from build123d import *

# Parameters (mm, degrees)
ESBO_O1_W                = 95.625
ESBO_O1_H                = 63.75
RESSALTO_EXTRUS_O1_DEPTH = 50
RESSALTO_EXTRUS_O2_DEPTH = 100
CORTE_EXTRUS_O1_DEPTH    = 100
CORTE_EXTRUS_O2_DEPTH    = 169
RESSALTO_EXTRUS_O3_DEPTH = 5


with BuildPart() as part:
    # Esboço1 → Ressalto-extrusão1 (new body)
    with BuildSketch(Plane.XY):
        with BuildLine():
            Line((0, 0), (0, -110))
            ThreePointArc((0, -110), (60, -134.792027106), (120, -110))
            Line((120, -110), (120, 0))
            ThreePointArc((120, 0), (60, 24.792027106), (0, 0))
        make_face()
        with Locations((60, -55)):
            Rectangle(ESBO_O1_W, ESBO_O1_H, mode=Mode.SUBTRACT)
    extrude(amount=RESSALTO_EXTRUS_O1_DEPTH)

    # Esboço2 → Ressalto-extrusão2 (add)
    with BuildSketch(Plane(origin=(0, 0, 0), x_dir=(-1, 0, 0), z_dir=(0, 0, -1))):
        with BuildLine():
            Line((-125, 2.041525096), (-125, -112.041525096))
            ThreePointArc((-125, -112.041525096), (-60, -139.792027106), (5, -112.041525096))
            Line((5, -112.041525096), (5, 2.041525096))
            ThreePointArc((5, 2.041525096), (-60, 29.792027106), (-125, 2.041525096))
        make_face()
        with BuildLine():
            Line((0, 0), (0, -110))
            ThreePointArc((0, -110), (-60, -134.792027106), (-120, -110))
            Line((-120, -110), (-120, 0))
            ThreePointArc((-120, 0), (-60, 24.792027106), (0, 0))
        make_face(mode=Mode.SUBTRACT)
    extrude(amount=-RESSALTO_EXTRUS_O2_DEPTH)

    # Esboço3 → Corte-extrusão1 (cut)
    with BuildSketch(Plane.XY.offset(50)):
        with BuildLine():
            Line((0, 0), (0, -110))
            ThreePointArc((0, -110), (60, -134.792027106), (120, -110))
            Line((120, -110), (120, 0))
            ThreePointArc((120, 0), (60, 24.792027106), (0, 0))
        make_face()
    extrude(amount=-CORTE_EXTRUS_O1_DEPTH, mode=Mode.SUBTRACT)

    # Esboço4 → Corte-extrusão2 (cut)
    with BuildSketch(Plane(origin=(125, 0, 0), x_dir=(0, 0, -1), z_dir=(1, 0, 0))):
        Polygon((-50, -55), (-100, -17.994062777), (-100, -175.493521459), (-50, -175.493521459), align=None)
    extrude(amount=-CORTE_EXTRUS_O2_DEPTH, mode=Mode.SUBTRACT)

    # Esboço5 → Ressalto-extrusão3 (add)
    with BuildSketch(Plane(origin=(0, 0, 0), x_dir=(-1, 0, 0), z_dir=(0, 0, -1))):
        with BuildLine():
            Line((-125, 2.041525096), (-125, -112.041525096))
            ThreePointArc((-125, -112.041525096), (-60, -139.792027106), (5, -112.041525096))
            Line((5, -112.041525096), (5, 2.041525096))
            ThreePointArc((5, 2.041525096), (-60, 29.792027106), (-125, 2.041525096))
        make_face()
        with BuildLine():
            Line((-116, -1.68447334), (-116, -108.31552666))
            ThreePointArc((-116, -108.31552666), (-60, -130.792027106), (-4, -108.31552666))
            Line((-4, -108.31552666), (-4, -1.68447334))
            ThreePointArc((-4, -1.68447334), (-60, 20.792027106), (-116, -1.68447334))
        make_face(mode=Mode.SUBTRACT)
    extrude(amount=RESSALTO_EXTRUS_O3_DEPTH)


solid = part.part
Build history of the part. All positions in model axes, mm. A direction names the side the tool comes from. Round coordinates to 2 decimals unless told otherwise and drop trailing zeros. Write each loop counter-clockwise with the first axis right and the second up, starting at its lowest first coordinate (ties: lowest second). Pieces come first, ordered by that corner, then holes. Notation, with made-up numbers: M 24.5,43 L 38.5,43 A32 cw 38.5,70 Z; hole C -26.5,-22.75 d4. An arc over 180 degrees is marked long. Answer in a Markdown table with one row per item.
1. Saw through at C-C (x = 29.5). List the corners of the cut face in (y, z), and give its area (3 significant figures).
Geometry check:
| item | result |
|---|---|
| outline | M -134.47,-5 L -124.83,-5 L -124.83,0 L -129.13,0 L -129.13,50 L -134.47,50 Z; M 14.83,-5 L 24.47,-5 L 24.47,100 L 19.13,100 L 19.13,0 L 14.83,0 Z |
| area | 897 mm2 |
2. Flat gauge pins, fed straight in: P1, Ø4, axis at x = 29.5, z = 23, coming from the +Y side; P2, Ø8, axis at x = 12.5, z = 56.5, coming from the +Y side. Where does each tip first touch, or does it go through?
Geometry check:
| item | result |
|---|---|
| P1 | y = 25.16 |
| P2 | y = 18.58 |
3. Mould opens along Y. For faces 1 (the face through (0, -42, 40)), 2 (the face through (118, -55, -5)), 3 (the face through (120, -44, 40)), 4 (the face through (58.983, 29.786, 48.235)) say: +Y half, -Y half, draft (parallel to the pull), parting line (faces both ways), or undercut.
Geometry check:
| item | result |
|---|---|
| face 1 | undercut |
| face 2 | draft |
| face 3 | undercut |
| face 4 | +Y half |
4. Saw through at B-B (z = 20). List the corners of the cut face in (x, y), and give its area (3 significant figures).
Geometry check:
| item | result |
|---|---|
| outline | M -5,-112.04 A90 ccw 125,-112.04 L 125,2.04 A90 ccw -5,2.04 Z; hole M 0,-110 A85 ccw 120,-110 L 120,0 A85 ccw 0,0 Z |
| area | 2,510 mm2 |
5. Saw through at D-D (z = 90.5). List the corners of the cut face in (x, y).
Geometry check:
| item | result |
|---|---|
| outline | M -5,-25.03 L 0,-25.03 L 0,0 A85 cw 120,0 L 120,-25.03 L 125,-25.03 L 125,2.04 A90 ccw -5,2.04 Z |
6. Which spindle directions (+Z, -Z, +X, -X, +Y, -Y) get a long thin tool onto all of the face, cutting with end or side? Do faces 5 (the face through (60, -135, 50)), 6 (the face through (60.866, -130.787, -2.465)), 7 (the face through (60.933, 24.787, 50.7)). Say none if no direction does.
Geometry check:
| item | result |
|---|---|
| face 5 | +Z, +X, -X, -Y |
| face 6 | +Z, -Z |
| face 7 | +Z |
7. Saw through at A-A (y = -16). List the corners of the cut face in (x, z), and give its area (3 significant figures).
Geometry check:
| item | result |
|---|---|
| outline | M -5,-5 L 4,-5 L 4,0 L 0,0 L 0,100 L -5,100 Z; M 116,-5 L 125,-5 L 125,100 L 120,100 L 120,0 L 116,0 Z |
| area | 1,090 mm2 |
8. Probe L1, parallel to Y at x = 60.5, z = 26.5; L2, parallel to X at y = -106.5, z = 48; L3, parallel to X at y = 15, z = 38. List the from-to ranges inside material, lowest first. Write a range as [from, to].
Geometry check:
| item | result |
|---|---|
| L1 | [-139.79, -134.79], [24.79, 29.79] |
| L2 | [-5, 0], [120, 125] |
| L3 | [10.57, 20.39], [99.61, 109.43] |
